Here's how the part is built. I have some questions about the finished solid (model axes, mm). A direction names the side the tool comes from. Give positions to 0.01 mm unless a question says otherwise; leave off trailing zeros. Loops run counter-clockwise (first coordinate to the right, second up) from the corner with the lowest first, then second, coordinate; pieces in that order, holes last. Notation, with made-up numbers: (76.25, 5.25) - (127.25, 5.25) arc R30 ccw to (127.25, 31.25) - close; hole circle Ø4 at (-27, 31.5). An arc over 180 degrees is marked (long way). Return JSON: item names as keys, results as strings. Group by question number.
(1) On a 3-axis mill with a long thin cutter (end or side, diameter ignored), from which of +Z, -Z, +X, -X, +Y, -Y can I reach the whole of each face in a straight line? I mean faces 1 (the flat face through (8, -25, 30)), 2 (the flat face through (0, 0, 0)), 3 (the cylindrical face through (23.846, 7.509, 14.79)), 4 (the flat face through (0, 10, 30)). Say none if no direction works.
(2) If we section it at D-D (z = 13): Please give me the cut outline in (x, y), then the cut area to 3 significant figures.
(3) For P1, Ø2, axis at x = -1, z = 28, coming from the +Y side; P2, Ø4, axis at x = -16, y = 15.5, coming from the +Z side; P3, Ø6, axis at y = -25, z = 13, coming from the -X side, each with a flat end and sliding along its axis, tell me the tip position at first contact or that it passes through.
(4) If we section it at B-B (y = -5.5): Please give me the cut outline in (x, z).
(5) If we section it at A-A (x = 0): Please give me the cut outline in (y, z).
(6) If we section it at C-C (z = 31): Please give me the cut outline in (x, y), then the cut area to 3 significant figures.
(7) I need wall thicknesses on probe 1 along Y at (x, z) = (-0.5, 38); probe 2 along Z at (x, y) = (24.5, -20.5); probe 3 along X at (y, z) = (19.5, 16.5). Which ranges of each line are inside material? Lowest first, please. Write a range as [from, to].
```python
from build123d import *

# Parameters (mm, degrees)
SKETCH1_R           = 25
BOSS_EXTRUDE1_DEPTH = 30
BOSS_EXTRUDE2_DEPTH = 10


with BuildPart() as part:
    # Sketch1 → Boss-Extrude1 (new body)
    with BuildSketch(Plane.XY):
        Circle(SKETCH1_R)
    extrude(amount=BOSS_EXTRUDE1_DEPTH)

    # Sketch2 → Boss-Extrude2 (add)
    with BuildSketch(Plane.XY.offset(30)):
        with BuildLine():
            Line((-35, 0), (35, 0))
            ThreePointArc((35, 0), (0, -35), (-35, 0))
        make_face()
    extrude(amount=BOSS_EXTRUDE2_DEPTH)


solid = part.part
```
Values:
{
 "1": {"face 1": "-Z, -Y", "face 2": "-Z, +X, -X, +Y, -Y", "face 3": "-Z", "face 4": "+Z, +X, -X, +Y"},
 "2": {"outline": "circle Ø50 at (0, 0)", "area": "1,960 mm2"},
 "3": {"P1": "y = 25", "P2": "z = 30", "P3": "x = -11.87"},
 "4": {"outline": "(-34.57, 30) - (-24.39, 30) - (-24.39, 0) - (24.39, 0) - (24.39, 30) - (34.57, 30) - (34.57, 40) - (-34.57, 40) - close"},
 "5": {"outline": "(-35, 30) - (-25, 30) - (-25, 0) - (25, 0) - (25, 30) - (0, 30) - (0, 40) - (-35, 40) - close"},
 "6": {"outline": "(-35, 0) arc R35 ccw to (35, 0) - close", "area": "1,920 mm2"},
 "7": {"probe 1": "[-35, 0]", "probe 2": "[30, 40]", "probe 3": "[-15.64, 15.64]"}
}
